from build123d import *

# Parameters (mm, degrees)
F0_W     = 76.2
F0_H     = 25.4
F1_DEPTH = 25.4
F2_W     = 25.4
F2_H     = 25.4
F3_DEPTH = 25.4
F4_W     = 25.4
F4_H     = 25.4
F5_DEPTH = 25.4
F6_W     = 25.4
F6_H     = 25.4
F7_DEPTH = 25.4


with BuildPart() as f1:
    # F0 (on Front) → F1 (new body)
    with BuildSketch(Plane.XZ):
        with Locations((5.309489, -4.486644)):
            Rectangle(F0_W, F0_H)
    extrude(amount=F1_DEPTH)

    # F2 (on face) → F3 (join)
    with BuildSketch(Plane(origin=(0, 0, 0), x_dir=(-1, 0, 0), z_dir=(0, 1, 0))):
        with Locations((-30.709489, -4.486644)):
            Rectangle(F2_W, F2_H)
    extrude(amount=F3_DEPTH)

    # F4 (on face) → F5 (join)
    with BuildSketch(Plane.XY.offset(8.213356)):
        with Locations((-20.090511, -12.7)):
            Rectangle(F4_W, F4_H)
    extrude(amount=F5_DEPTH)

    # F6 (on face) → F7 (join)
    with BuildSketch(Plane.XZ.offset(25.4)):
        with Locations((-20.090511, 20.913356)):
            Rectangle(F6_W, F6_H)
    extrude(amount=F7_DEPTH)


solid = f1.part
The listing builds one solid part. Answer for the finished solid, in the listing's coordinates (mm). A direction names the side the tool comes from. Give positions to 0.01 mm unless a question says otherwise; leave off trailing zeros. Loops run counter-clockwise (first coordinate to the right, second up) from the corner with the lowest first, then second, coordinate; pieces in that order, holes last. Notation, with made-up numbers: (82.25, 51) - (88.25, 51) arc R28 ccw to (88.25, 87) - close; hole circle Ø6 at (87, 8.5). An arc over 180 degrees is marked (long way). Use one line per item in the form item = value.
1. Section D-D on z = 30 is taken. Give the vertices of the cut face in (x, y), then the cut area to 3 significant figures.
Calculated:
outline = (-32.79, -50.8) - (-7.39, -50.8) - (-7.39, 0) - (-32.79, 0) - close
area = 1,290 mm^2
2. Section A-A on z = 0.5 is taken. Give the vertices of the cut face in (x, y).
Calculated:
outline = (-32.79, -25.4) - (43.41, -25.4) - (43.41, 25.4) - (18.01, 25.4) - (18.01, 0) - (-32.79, 0) - close
3. Find the intervals of material crossed by line 1 along Y through (x, z) = (-12, -11.5); line 2 along Z through (x, y) = (-3.5, -20.5); line 3 along Y through (x, z) = (22.5, -6.5), in increasing order. Write a range as [from, to].
Calculated:
line_1 = [-25.4, 0]
line_2 = [-17.19, 8.21]
line_3 = [-25.4, 25.4]
4. Which of the six approach directions +Z, -Z, +X, -X, +Y, -Y give full straight-line access (tool end or side, diameter ignored) to faces 1 (the face through (-20, -50.8, 21)), 2 (the face through (5, -25.4, -5)), 3 (the face through (31, 25.4, -4)), 4 (the face through (24, -6, 8.213)), 5 (the face through (-13, 0, 2))?
Calculated:
face_1 = +Z, -Z, +X, -X, -Y
face_2 = -Z, +X, -X, -Y
face_3 = +Z, -Z, +X, -X, +Y
face_4 = +Z, +X, +Y, -Y
face_5 = +Z, -Z, -X, +Y
5. The mould has two halves that part along Z. Classify faces 6 (the face through (-20, -25, 33.613)), 7 (the face through (-20, -38, 8.213)), 8 (the face through (43.409, 0, -5)): pulls with the +Z half, pulls with the -Z half, needs draft (parallel to the pull), parting line crosses it, or undercut.
Calculated:
face_6 = pulls with the +Z half
face_7 = pulls with the -Z half
face_8 = needs draft
6. Section C-C on y = 18.5 is taken. Give the vertices of the cut face in (x, z).
Calculated:
outline = (18.01, -17.19) - (43.41, -17.19) - (43.41, 8.21) - (18.01, 8.21) - close
7. Section B-B on x = -14 is taken. Give the vertices of the cut face in (y, z), then the cut area to 3 significant figures.
Calculated:
outline = (-50.8, 8.21) - (-25.4, 8.21) - (-25.4, -17.19) - (0, -17.19) - (0, 33.61) - (-50.8, 33.61) - close
area = 1,940 mm^2
8. Given pin 1 Ø7.5 at (x, z) = (-4.5, -7) entering from -Y; pin 2 Ø7.5 at (x, y) = (-21, -44) entering from -Z; pin 3 Ø3 at (y, z) = (-30, 17) entering from +X, each flat-ended and moving along its own axis, determine where each tip first touches the part or whether it passes through.
Calculated:
pin_1 = -25.4
pin_2 = 8.21
pin_3 = -7.39
